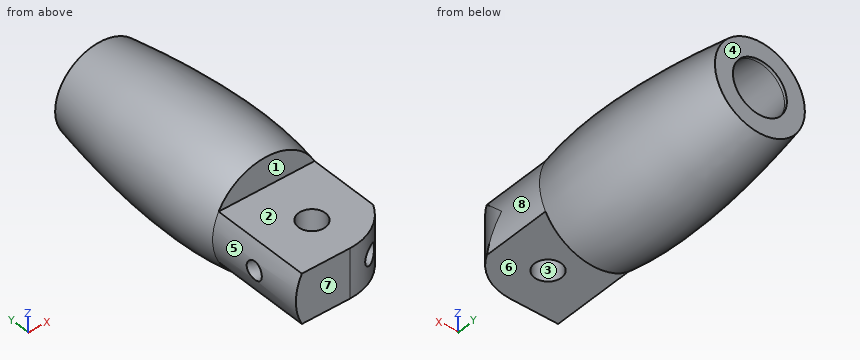
from build123d import *

# Parameters (mm, degrees)
BOSS_EXTRUDE1_DEPTH     = 2.75
CUT_EXTRUDE5_DEPTH      = 14
CUT_EXTRUDE5_DEPTH_BACK = 14
SKETCH5_R               = 1.5
SKETCH6_OUTSIDE_W       = 22.626
SKETCH6_OUTSIDE_H       = 22.626
SKETCH6_OUTSIDE_R       = 6
CUT_EXTRUDE6_DEPTH      = 24.860169667
SKETCH7_R               = 1
CUT_EXTRUDE7_DEPTH      = 20
SKETCH8_R               = 1


with BuildPart() as part:
    # Sketch1 → Revolve1 (revolve)
    with BuildSketch(Plane(origin=(0, 0, 0), x_dir=(0, 0, -1), z_dir=(1, 0, 0))):
        with BuildLine():
            Line((0, 2), (0, 0))
            Line((0, 0), (6, 0))
            add(Edge.make_bspline(
                [(5, 22), (7.432624423, 8.203901334), (6, 0)],
                knots=[0, 0, 0, 1, 1, 1], degree=2))
            Line((5, 22), (3, 22))
            add(Edge.make_bspline(
                [(3.030384494, 21.652703645), (3.016873864, 21.729326237), (3, 22)],
                knots=[0, 0, 0, 1, 1, 1], degree=2))
            add(Edge.make_bspline(
                [(3.030384494, 21.652703645), (3.725648232, 17.709667047), (4.838461357, 7.341433009), (4.295069583, 2.215324441), (4.269810085, 2)],
                knots=[0, 0, 0, 0.289998028, 0.869994084, 0.895995268, 0.895995268, 0.895995268], degree=2))
            Line((4.269810085, 2), (0, 2))
        make_face()
    revolve(axis=Axis((0, 0, 0), (0, 1, 0)))

    # Sketch3 → Boss-Extrude1 (add, symmetric)
    with BuildSketch(Plane.XY):
        with BuildLine():
            Line((-6, 0), (-6, -11))
            Line((-6, -11), (0, -11))
            ThreePointArc((0, -11), (4.242640687, -9.242640687), (6, -5))
            Line((6, -5), (6, 0))
            Line((6, 0), (-6, 0))
        make_face()
    extrude(amount=BOSS_EXTRUDE1_DEPTH, both=True)

    # Sketch5 → Cut-Extrude5 (cut, two sides: drawn at the far end of the back side and taken through both)
    with BuildSketch(Plane.XY.offset(-CUT_EXTRUDE5_DEPTH_BACK)):
        with Locations((0, -6)):
            Circle(SKETCH5_R)
    extrude(amount=CUT_EXTRUDE5_DEPTH + CUT_EXTRUDE5_DEPTH_BACK, mode=Mode.SUBTRACT)

    # Sketch6 outside → Cut-Extrude6 (cut, through all)
    with BuildSketch(Plane(origin=(0, 0, 0), x_dir=(1, 0, 0), z_dir=(0, 1, 0))):
        Rectangle(SKETCH6_OUTSIDE_W, SKETCH6_OUTSIDE_H)
        Circle(SKETCH6_OUTSIDE_R, mode=Mode.SUBTRACT)
    extrude(amount=-CUT_EXTRUDE6_DEPTH, mode=Mode.SUBTRACT)

    # Sketch7 → Cut-Extrude7 (cut)
    with BuildSketch(Plane.XZ.offset(11)):
        with Locations(Location((3, 0, 0), (0, 0, 270))):
            Circle(SKETCH7_R)
    extrude(amount=-CUT_EXTRUDE7_DEPTH, mode=Mode.SUBTRACT)

    # Cut-Sweep1: sweep along a path in Sketch10
    with BuildLine() as cut_sweep1_path:  # in the path sketch's own coordinates; laid on its plane below (add() does not lay a ready-made edge on the line's plane)
        add(Edge.make_bspline(
            [(-6, -5.5), (-2.332682252, -5.5), (-2.332682252, 2)],
            knots=[0, 0, 0, 1, 1, 1], degree=2))
    # Sketch8 → Cut-Sweep1 (sweep, cut)
    with BuildSketch(Plane.ZY.offset(6)):
        with Locations((0, -5.5)):
            Circle(SKETCH8_R)
    sweep(path=Plane.XY * cut_sweep1_path.line, mode=Mode.SUBTRACT)


solid = part.part
Model file for the job. Use its own axes, mm. Face numbers are marked on the shaded views. A direction names the side the tool comes from. Give positions to 0.01 mm unless a question says otherwise; leave off trailing zeros.
Item 1: Mould opens along Y. For the marked faces 1, 2 and 3 say: +Y half, -Y half, draft (parallel to the pull), parting line (faces both ways), or undercut.
Check values:
face 1: -Y half
face 2: draft
face 3: undercut
Item 2: Slice it at A-A (y = -6). Give the number of separate pieces and of enclosed holes in the cut face, plus the area to 3 significant figures.
Check values:
separate pieces: 2
enclosed holes: 1
area: 41.1 mm2
Item 3: Drop flat-ended pins along their axis: P1, Ø4, axis at x = 0, y = -6, coming from the +Z side; P2, Ø5, axis at y = 13, z = 4.5, coming from the +X side; P3, Ø6, axis at x = 4, z = 3.5, coming from the -Y side. Give the stop position or say it passes through.
Check values:
P1: stops at z = 2.75
P2: stops at x = 5.93
P3: stops at y = -10.9
Item 4: Drill centre lines: line 1 along Z through (x, y) = (3, -1); line 2 along X through (y, z) = (-0.25, 0); line 3 along X through (y, z) = (-6, 0.05). Where is each one in solid material? Low to high.
Check values:
line 1: z = -2.75 to -1, 1 to 2.75
line 2: x = -6 to -3.44, -1.43 to 2, 4 to 6
line 3: x = -4.06 to -1.5, 1.5 to 2, 4 to 5.92
Item 5: Which spindle directions (+Z, -Z, +X, -X, +Y, -Y) get a long thin tool onto all of the face, cutting with end or side? Do the marked faces 4, 5, 6, 7 and 8. Say none if no direction does.
Check values:
face 4: +Z, -Z, +X, -X, +Y
face 5: -X, -Y
face 6: -Z, +X, -X, -Y
face 7: +Z, -Z, +X, -X, -Y
face 8: +X, -Y
